from build123d import *

# Parameters (mm, degrees)
F0_R     = 23
F0_R_2   = 20
F1_DEPTH = 15
F2_R     = 23
F3_DEPTH = 3
F4_R     = 1


with BuildPart() as f1:
    # F0 (on Top) → F1 (new body)
    with BuildSketch(Plane.XY):
        Circle(F0_R)
        Circle(F0_R_2, mode=Mode.SUBTRACT)
    extrude(amount=F1_DEPTH)

    # F2 (on Top) → F3 (join)
    with BuildSketch(Plane.XY):
        Circle(F2_R)
    extrude(amount=-F3_DEPTH)

    # F4
    f4_edges = [f1.edges().sort_by_distance(p)[0] for p in [
        (-23, 0, 15),
        (-20, 0, 15),
        (23, 0, 7.5),
        (-23, 0, 0),
    ]]
    fillet(f4_edges, radius=F4_R)


solid = f1.part
Here's how the part is built. I have some questions about the finished solid (model axes, mm). Give positions to 0.01 mm unless a question says otherwise; leave off trailing zeros. Order: outer loops, then holes, each group sorted by start corner. A loop starts at its lowest first (then second) coordinate and runs counter-clockwise, first axis right, second up. Notation, with made-up numbers: M 7,80.25 L 11,80.25 A18 ccw 11,92.25 Z; hole C 79,77 d1. An arc over 180 degrees is marked long. Answer as a JSON object with one key per item and string values. Group by question number.
1) I'm going to push flat-ended pins straight in: pin 1 Ø1 at (y, z) = (11.5, 0.5) entering from -X; pin 2 Ø4 at (x, y) = (-6, 15.5) entering from +Z; pin 3 Ø6 at (x, z) = (-17, 3.5) entering from -Y; pin 4 Ø10 at (y, z) = (-2, 6) entering from -X. Where does each tip first touch, or does it pass through?
2) We'd pull the mould along Y, two halves only. Please class faces 1 (the cylindrical face through (-4.336, -19.524, 6.902)), 2 (the cylindrical face through (-2.994, 22.804, 6.112)), 3 (the flat face through (0, 0, -3)): pulls with the +Y half, pulls with the -Y half, needs draft (parallel to the pull), parting line crosses it, or undercut.
3) Please list where these lines run through material, in increasing order: L1, parallel to Y at x = 0, z = 3.5; L2, parallel to Z at x = -7.5, y = -9.5; L3, parallel to Y at x = 13, z = 2.5. Write a range as [from, to].
4) Suppose I cut it at A-A, the plane z = 1.25. Write out the boundary of the cut face in (x, y), plus the area to 3 significant figures.
5) Suppose I cut it at B-B, the plane y = 0. Write out the boundary of the cut face in (x, z), plus the area to 3 significant figures.
Results found:
{
 "1": {"pin 1": "x = -20.2", "pin 2": "z = 0", "pin 3": "y = -18.25", "pin 4": "x = -23"},
 "2": {"face 1": "undercut", "face 2": "parting line crosses it", "face 3": "needs draft"},
 "3": {"L1": "[-23, -20], [20, 23]", "L2": "[-3, 0]", "L3": "[-18.97, -15.2], [15.2, 18.97]"},
 "4": {"outline": "C 0,0 d46; hole C 0,0 d40", "area": "405 mm²"},
 "5": {"outline": "M -23,-2 A1 ccw -22,-3 L 22,-3 A1 ccw 23,-2 L 23,14 A1 ccw 22,15 L 21,15 A1 ccw 20,14 L 20,0 L -20,0 L -20,14 A1 ccw -21,15 L -22,15 A1 ccw -23,14 Z", "area": "227 mm²"}
}
